CAD build for the part. Positions are in the model's coordinates, mm. A direction names the side the tool comes from. Round coordinates to 2 decimals unless told otherwise and drop trailing zeros. Loops run counter-clockwise (first coordinate to the right, second up) from the corner with the lowest first, then second, coordinate; pieces in that order, holes last. Notation, with made-up numbers: (-30.5, 13) -> (26.5, 13) arc R16 cw to (26.5, 30) -> close; hole circle Ø11 at (10.25, 5). An arc over 180 degrees is marked (long way). Answer as CSV lines item,"result".
```python
from build123d import *

# Parameters (mm, degrees)
SKETCH1_R           = 2.3
SKETCH1_W           = 19
SKETCH1_H           = 10
BOSS_EXTRUDE1_DEPTH = 22
BOSS_EXTRUDE2_REACH = 39.9
SKETCH5_R           = 2.6
CUT_EXTRUDE1_DEPTH  = 17.5


with BuildPart() as part:
    # Sketch1 → Boss-Extrude1 (new body)
    with BuildSketch(Plane(origin=(0, 0, 0), x_dir=(1, 0, 0), z_dir=(0, 1, 0))):
        with BuildLine():
            Line((-32, 0), (-32, -27.5))
            ThreePointArc((-32, -27.5), (-30.096194078, -32.096194078), (-25.5, -34))
            Line((-25.5, -34), (-6.5, -34))
            ThreePointArc((-6.5, -34), (-1.903805922, -32.096194078), (0, -27.5))
            Line((0, -27.5), (0, 0))
            Line((0, 0), (-3.25, 0))
            Line((-3.25, 0), (-3.25, 2.3))
            Line((-3.25, 2.3), (-0.225, 2.3))
            Line((-0.225, 2.3), (-0.225, 3))
            Line((-0.225, 3), (-3.25, 5.9))
            Line((-3.25, 5.9), (-8.75, 5.9))
            Line((-8.75, 5.9), (-11.775, 3))
            Line((-11.775, 3), (-11.775, 2.3))
            Line((-11.775, 2.3), (-8.75, 2.3))
            Line((-8.75, 2.3), (-8.75, 0))
            Line((-8.75, 0), (-23.25, 0))
            Line((-23.25, 0), (-23.25, 2.3))
            Line((-23.25, 2.3), (-20.225, 2.3))
            Line((-20.225, 2.3), (-20.225, 3))
            Line((-20.225, 3), (-23.25, 5.9))
            Line((-23.25, 5.9), (-28.75, 5.9))
            Line((-28.75, 5.9), (-31.775, 3))
            Line((-31.775, 3), (-31.775, 2.3))
            Line((-31.775, 2.3), (-28.75, 2.3))
            Line((-28.75, 2.3), (-28.75, 0))
            Line((-28.75, 0), (-32, 0))
        make_face()
        with Locations((-16, -7)):
            Circle(SKETCH1_R, mode=Mode.SUBTRACT)
        with Locations((-16, -27)):
            Rectangle(SKETCH1_W, SKETCH1_H, mode=Mode.SUBTRACT)
    extrude(amount=BOSS_EXTRUDE1_DEPTH)

    # Sketch2 → Boss-Extrude2 (add, up to next)
    with BuildSketch(Plane(origin=(0, 0, 32), x_dir=(-1, 0, 0), z_dir=(0, 0, -1)), mode=Mode.PRIVATE) as boss_extrude2_sk1:
        with BuildLine():
            Line((21.5, 0), (21.5, 8.519259302))
            ThreePointArc((21.5, 8.519259302), (16, 6.5), (10.5, 8.519259302))
            Line((10.5, 8.519259302), (10.5, 0))
            Line((10.5, 0), (21.5, 0))
        make_face()
    boss_extrude2_tool1 = extrude(boss_extrude2_sk1.sketch, amount=BOSS_EXTRUDE2_REACH, mode=Mode.PRIVATE) - part.part
    add(boss_extrude2_tool1.solids().sort_by_distance((-16, 3.593056, 32))[0])

    # Sketch4 → Revolve1 (revolve)
    with BuildSketch(Plane(origin=(-16, 0, 0), x_dir=(0, 0, -1), z_dir=(1, 0, 0))):
        Polygon((-32, 20), (-31.1, 18.5), (-31.1, 15), (-32, 15), align=None)
        Polygon((-22, 15), (-22.9, 15), (-22.9, 18.5), (-22, 20), align=None)
    revolve(axis=Axis((-16, 15, 32), (0, 0, -1)))

    # Sketch5 → Cut-Extrude1 (cut)
    with BuildSketch(Plane.XY.offset(34)):
        with Locations((-16, 15)):
            Circle(SKETCH5_R)
    extrude(amount=-CUT_EXTRUDE1_DEPTH, mode=Mode.SUBTRACT)


solid = part.part
```
Q1. Probe L1, parallel to Z at x = -22.5, y = 17.5; L2, parallel to Y at x = -16, z = 20.5; L3, parallel to Z at x = -25, y = 14.5. List the from-to ranges inside material, lowest first. Write a range as [from, to].
Results:
L1,"[-5.18, -2.3], [0, 22], [32, 34]"
L2,"[0, 12.4], [17.6, 22]"
L3,"[-5.9, 22], [32, 34]"
Q2. Drop flat-ended pins along their axis: pin 1 Ø4 at (x, y) = (-21, 9.5) entering from -Z; pin 2 Ø1.2 at (y, z) = (6, -1) entering from +X; pin 3 Ø5 at (x, z) = (-6.5, 5.5) entering from -Y; pin 4 Ø2 at (x, y) = (-18.5, 10.5) entering from -Z. Give the stop position or say it passes through.
Results:
pin 1,"z = -5.66"
pin 2,"x = -3.25"
pin 3,"y = 0"
pin 4,"z = 0"
Q3. Slice it at B-B, the plane z = -1. Give the cut face in (x, y), and give its area (3 significant figures).
Results:
outline,"(-28.75, 0) -> (-23.25, 0) -> (-23.25, 22) -> (-28.75, 22) -> close; (-8.75, 0) -> (-3.25, 0) -> (-3.25, 22) -> (-8.75, 22) -> close"
area,"242 mm2"
Q4. Slice it at D-D, the plane y = 20.5. Count the separate pieces of the cut face and the enclosed holes in it, and give its area (3 significant figures).
Results:
separate pieces,"1"
enclosed holes,"2"
area,"954 mm2"
Q5. Tool access for faces 1 (the flat face through (-30, 11, -2.3)), 2 (the flat face through (-16, 8, 32)), 3 (the flat face through (-13, 15, 31.1)), 4 (the flat face through (-3.25, 11, -1)), 5 (the flat face through (-21.5, 4, 27)): list every direction of +Z, -Z, +X, -X, +Y, -Y with a clear straight run to the whole face (end or side of a thin tool).
Results:
face 1,"-X, +Y, -Y"
face 2,"none"
face 3,"+Y"
face 4,"+X, +Y, -Y"
face 5,"+Y, -Y"
Q6. Slice it at C-C, the plane z = 23.5. Give the cut face in (x, y).
Results:
outline,"(-32, 0) -> (-25.5, 0) -> (-25.5, 22) -> (-32, 22) -> close; (-21.5, 0) -> (-10.5, 0) -> (-10.5, 8.52) arc R8.5 cw to (-21.5, 8.52) -> close; (-6.5, 0) -> (0, 0) -> (0, 22) -> (-6.5, 22) -> close"
Q7. Two-plate mould, pull along Z, no slides. Class faces 6 (the cylindrical face through (-1.955, 10.846, 32.146)), 7 (the flat face through (-16, 22, 14)), 8 (the flat face through (-10, 11, -2.3)): pulls with the +Z half, pulls with the -Z half, needs draft (parallel to the pull), parting line crosses it, or undercut.
Results:
face 6,"pulls with the +Z half"
face 7,"needs draft"
face 8,"undercut"
Q8. Slice it at A-A, the plane x = -16. Give the cut face in (y, z).
Results:
outline,"(0, 0) -> (22, 0) -> (22, 4.7) -> (0, 4.7) -> close; (0, 9.3) -> (22, 9.3) -> (22, 22) -> (20, 22) -> (18.5, 22.9) -> (17.6, 22.9) -> (17.6, 16.5) -> (12.4, 16.5) -> (12.4, 22.9) -> (11.5, 22.9) -> (10, 22) -> (6.5, 22) -> (6.5, 32) -> (10, 32) -> (11.5, 31.1) -> (12.4, 31.1) -> (12.4, 34) -> (0, 34) -> close; (17.6, 31.1) -> (18.5, 31.1) -> (20, 32) -> (22, 32) -> (22, 34) -> (17.6, 34) -> close"
